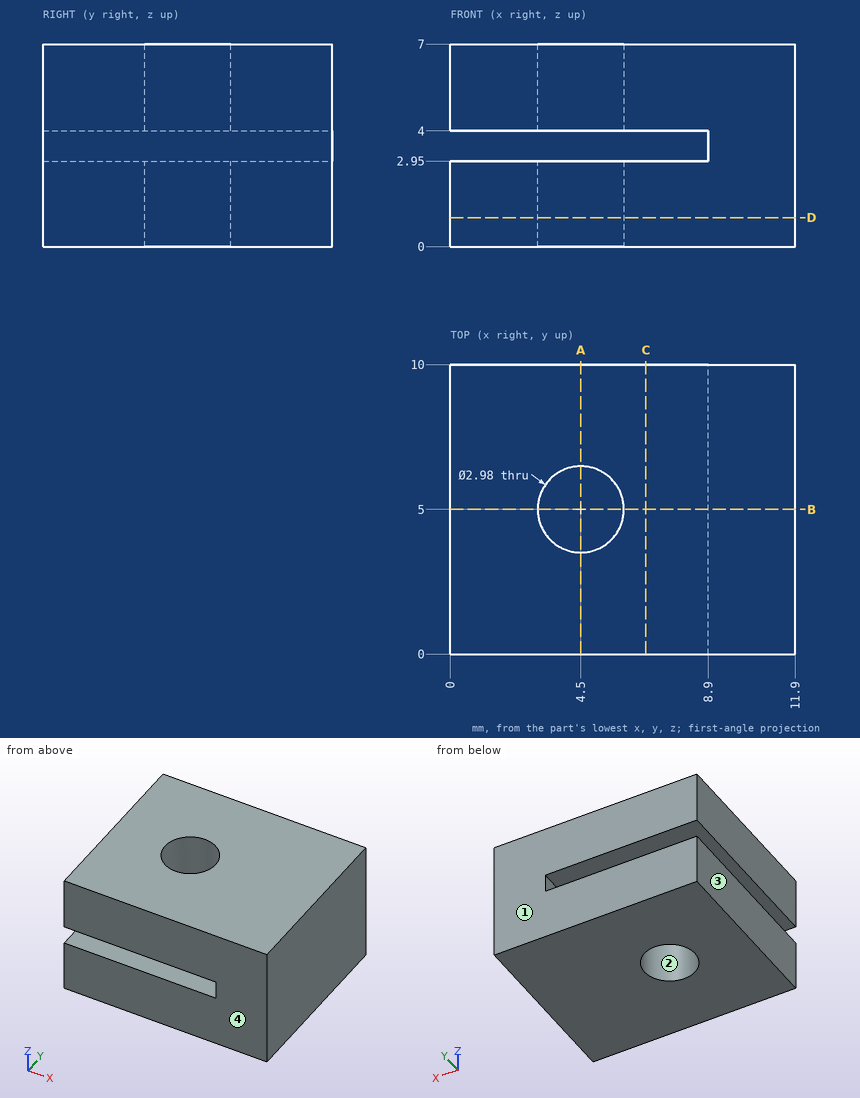
Answer from the drawing. Dimensions are ordinates in mm from the lowest x, y and z of the part. Give positions to 0.01 mm unless a question says otherwise; leave off trailing zeros. Loops run counter-clockwise (first coordinate to the right, second up) from the corner with the lowest first, then second, coordinate; pieces in that order, holes last. Notation, with made-up numbers: M 47.5,24 L 99.5,24 A7 ccw 99.5,36 Z; hole C 75.5,16.5 d2. An arc over 180 degrees is marked long. One line per item, written item: value.
Q1. A cutting plane is placed at D-D on z = 1. Determine the outline of the cut face in (x, y).
Working result:
outline: M 0,0 L 11.9,0 L 11.9,10 L 0,10 Z; hole C 4.5,5 d2.98
Q2. Find the intervals of material crossed by line 1 (Y direction, x = 4.5, z = 5.35); line 2 (Z direction, x = 7.5, y = 3); line 3 (X direction, y = 7, z = 3), in increasing order. Write a range as from..to.
Working result:
line 1: y = 0..3.51, 6.49..10
line 2: z = 0..2.95, 4..7
line 3: x = 8.9..11.9
Q3. A cutting plane is placed at B-B on y = 5. Determine the outline of the cut face in (x, z), then the cut area to 3 significant figures.
Working result:
outline: M 0,0 L 3.01,0 L 3.01,2.95 L 0,2.95 Z; M 0,4 L 3.01,4 L 3.01,7 L 0,7 Z; M 5.99,0 L 11.9,0 L 11.9,7 L 5.99,7 L 5.99,4 L 8.9,4 L 8.9,2.95 L 5.99,2.95 Z
area: 56.2 mm^2
Q4. Determine the mould class of the marked faces 1, 2, 3 and 4 for opening direction Y: +Y half, -Y half, draft (parallel to the pull), parting line (faces both ways), or undercut.
Working result:
face 1: +Y half
face 2: undercut
face 3: draft
face 4: -Y half
Q5. Flat-ended cylindrical pins translate along their axes: P1, Ø2.5, axis at x = 4, y = 6, coming from the +Z side; P2, Ø1.8, axis at x = 4.5, y = 5, coming from the -Z side; P3, Ø0.5, axis at y = 4, z = 3.5, coming from the -X side. Find the tip coordinate at first contact, or state that the pin passes through.
Working result:
P1: stops at z = 7
P2: passes through
P3: stops at x = 8.9
Q6. A cutting plane is placed at C-C on x = 6.75. Determine the outline of the cut face in (y, z), then the cut area to 3 significant figures.
Working result:
outline: M 0,0 L 10,0 L 10,2.95 L 0,2.95 Z; M 0,4 L 10,4 L 10,7 L 0,7 Z
area: 59.5 mm^2
Q7. A cutting plane is placed at A-A on x = 4.5. Determine the outline of the cut face in (y, z).
Working result:
outline: M 0,0 L 3.51,0 L 3.51,2.95 L 0,2.95 Z; M 0,4 L 3.51,4 L 3.51,7 L 0,7 Z; M 6.49,0 L 10,0 L 10,2.95 L 6.49,2.95 Z; M 6.49,4 L 10,4 L 10,7 L 6.49,7 Z
